```python
from build123d import *

# Parameters (mm, degrees)
SKETCH4_W = 10
SKETCH4_H = 10
FILLET1_R = 1
FILLET2_R = 1


with BuildPart() as part:
    # Sketch1 → Revolve1 (revolve)
    with BuildSketch(Plane(origin=(0, 0, 0), x_dir=(0, 0, -1), z_dir=(1, 0, 0)), mode=Mode.PRIVATE) as revolve1_sk:
        Polygon((0, 0), (8.5, 0), (4.821351766, 35), (0, 35), align=None)
    revolve(revolve1_sk.sketch.rotate(Axis((0, 13.119565217, 0), (0, -1, 0)), 180), axis=Axis((0, 13.119565217, 0), (0, -1, 0)))

    # Sweep1: sweep along a path in Sketch2
    with BuildLine(Plane.XY) as sweep1_path:
        Line((0, 35), (0, 42.002963953))
        ThreePointArc((0, 42.002963953), (2.984964946, 47.737028263), (9.394141003, 48.580812298))
        Line((9.394141003, 48.580812298), (18.793852416, 45.159597133))
    # Sketch4 → Sweep1 (sweep)
    with BuildSketch(Plane(origin=(2.081374564, -0.757558388, 0), x_dir=(0.3420201433256729, 0.9396926207859069, 0), z_dir=(0.9396926207859069, -0.3420201433256729, 0))):
        with Locations((48.864016281, 0)):
            Rectangle(SKETCH4_W, SKETCH4_H)
    sweep(path=sweep1_path.line)

    # Fillet1
    fillet1_edges = [part.edges().sort_by_distance(p)[0] for p in [
        (-5, 38.501481976, -5),
        (-5, 38.501481976, 5),
        (0.117082764, 51.832788484, -5),
        (0.117082764, 51.832788484, 5),
        (15.804097426, 51.56866782, -5),
        (15.804097426, 51.56866782, 5),
    ]]
    fillet(fillet1_edges, radius=FILLET1_R)

    # Fillet2
    fillet2_edges = [part.edges().sort_by_distance(p)[0] for p in [
        (5, 38.501481976, -5),
        (5, 38.501481976, 5),
        (5.852847127, 43.641268041, -5),
        (5.852847127, 43.641268041, 5),
        (12.383895993, 42.171741612, -5),
        (12.383895993, 42.171741612, 5),
    ]]
    fillet(fillet2_edges, radius=FILLET2_R)


solid = part.part
```
Geometry: final body of the model. Coordinates: model frame, mm. A direction names the side the tool comes from. Give positions to 0.01 mm unless a question says otherwise; leave off trailing zeros. Order: outer loops, then holes, each group sorted by start corner. A loop starts at its lowest first (then second) coordinate and runs counter-clockwise, first axis right, second up. Notation, with made-up numbers: (24, 71) -> (53, 71) arc R26 cw to (53, 110) -> close; hole circle Ø11 at (61.5, 21). An arc over 180 degrees is marked (long way). Write each question's results on one line, items separated by ' | '. Start each with the question number.
1) Section B-B (y = 6). Return loops of the section in (x, z), then the cut area to 3 significant figures.
2) Section C-C (y = 29). Return loops of the section in (x, z).
3) First-contact query: pin 1 (10 mm diameter, centred on y = 24, z = 6, fed in from +X); pin 2 (5.5 mm diameter, centred on y = 37.5, z = -1.5, fed in from +X); pin 3 (3 mm diameter, centred on y = 37.5, z = 2, fed in from -X); pin 4 (10 mm diameter, centred on x = 3, z = -1.5, fed in from -Y). Flat tips, straight axial feed; report the tip coordinate or a pass-through.
4) Draft query along Y for faces 5 (the flat face through (-5, 39, 0)), 6 (the cylindrical face through (5.831, 43.626, -0.056)), 7 (the flat face through (0, 0, 0)). Return one class per face: pulls with the +Y half, pulls with the -Y half, needs draft (parallel to the pull), parting line crosses it, or undercut.
5) Section A-A (z = 0). Return loops of the section in (x, y), then the cut area to 3 significant figures.
6) Set-up query: faces 1 (the cylindrical face through (12.547, 42.416, -4.699)), 2 (the flat face through (-4, 35, -3)), 3 (the cylindrical face through (-4.699, 38.551, 4.715)), 4 (the flat face through (5, 46, 5)). Return all of +Z, -Z, +X, -X, +Y, -Y with unobstructed straight access to the full face (end or side cutting, diameter ignored); none if empty.
7) Line query: line 1 (Z direction, x = 2.5, y = 51.5); line 2 (X direction, y = 22, z = 1.5). Output: solid intervals per line, ascending. Write a range as from..to.
Calculated:
1) outline: circle Ø15.74 at (0, 0) | area: 195 mm2
2) outline: circle Ø10.9 at (0, 0)
3) pin 1: x = 6.02 | pin 2: x = 5 | pin 3: x = -5 | pin 4: y = 0
4) face 5: needs draft | face 6: undercut | face 7: pulls with the -Y half
5) outline: (-8.5, 0) -> (8.5, 0) -> (4.82, 35) -> (5, 35) -> (5, 42) arc R2 cw to (7.68, 43.88) -> (17.08, 40.46) -> (20.5, 49.86) -> (11.1, 53.28) arc R12 ccw to (-5, 42) -> (-5, 35) -> (-4.82, 35) -> close | area: 771 mm2
6) face 1: -Z, -Y | face 2: none | face 3: +Z, -X, +Y | face 4: +Z, +X, -X, +Y
7) line 1: -5..5 | line 2: -6..6
